Check sheet for the modelled part. Datum: model origin and axes. Units: mm. A direction names the side the tool comes from. Give positions to 0.01 mm unless a question says otherwise; leave off trailing zeros. Write each loop counter-clockwise with the first axis right and the second up, starting at its lowest first coordinate (ties: lowest second). Pieces come first, ordered by that corner, then holes. Notation, with made-up numbers: (-32, -11) -> (-27, -11) arc R12 ccw to (-27, 7) -> close; hole circle Ø3 at (16, 38). An arc over 180 degrees is marked (long way). Return JSON: item names as keys, results as strings.
from build123d import *

# Parameters (mm, degrees)
F1_DEPTH  = 153.75
F2_SIZE   = 3
F3_R      = 3.1
F4_DEPTH  = 11.001
F6_DEPTH  = 7
F7_R      = 27
F8_DEPTH  = 18.67
F9_R      = 14.75
F10_DEPTH = 3
F12_W     = 1
F12_H     = 1
F14_R     = 7.5
F15_DEPTH = 18.5
F16_R     = 9.425
F16_R_2   = 7.5
F17_DEPTH = 13.08
F19_DEPTH = 16
F20_R     = 27.5
F21_DEPTH = 10


# Not quite as in the source:
# - the program builds the solid bodies; features that only make, move or delete a surface that nothing else refers to are left out


with BuildPart() as f1:
    # F0 (on Front) → F1 (new body)
    with BuildSketch(Plane.XZ):
        Polygon((0, 11), (0, 0), (94, 0), (94, 11), (82, 11), (82, 77), (12, 77), (12, 11), align=None)
    extrude(amount=F1_DEPTH)

    # F2
    f2_edges = [f1.edges().sort_by_distance(p)[0] for p in [
        (12, -76.875, 77),
        (82, -76.875, 77),
    ]]
    chamfer(f2_edges, length=F2_SIZE)

    # F3 (on face) → F4 (cut, through all)
    with BuildSketch(Plane.XY.offset(11)):
        with Locations((89, -133.75)):
            Circle(F3_R)
        with Locations((89, -95.65)):
            Circle(F3_R)
        with Locations((89, -57.55)):
            Circle(F3_R)
        with Locations((89, -19.45)):
            Circle(F3_R)
        with Locations((5, -19.45)):
            Circle(F3_R)
        with Locations((5, -57.55)):
            Circle(F3_R)
        with Locations((5, -95.65)):
            Circle(F3_R)
        with Locations((5, -133.75)):
            Circle(F3_R)
    extrude(amount=-F4_DEPTH, mode=Mode.SUBTRACT)

    # F5 (on face) → F6 (join)
    with BuildSketch(Plane.XZ.offset(153.75)):
        with BuildLine():
            Line((25.9310321962, 77), (25.9310321962, 62.0646068434))
            ThreePointArc((25.9310321962, 62.0646068434), (15.39, 38.5), (25.9310321962, 14.9353931566))
            Line((25.9310321962, 14.9353931566), (25.9310321962, 0))
            Line((25.9310321962, 0), (68.0689678038, 0))
            Line((68.0689678038, 0), (68.0689678038, 14.9353931566))
            ThreePointArc((68.0689678038, 14.9353931566), (78.61, 38.5), (68.0689678038, 62.0646068434))
            Line((68.0689678038, 62.0646068434), (68.0689678038, 77))
            Line((68.0689678038, 77), (25.9310321962, 77))
        make_face()
    extrude(amount=F6_DEPTH)

    # F7 (on face) → F8 (join)
    with BuildSketch(Plane.XZ.offset(160.75)):
        with Locations((47, 38.5)):
            Circle(F7_R)
    extrude(amount=F8_DEPTH)

    # F9 (on face) → F10 (join)
    with BuildSketch(Plane.XZ.offset(179.42)):
        with Locations((47, 38.5)):
            Circle(F9_R)
    extrude(amount=F10_DEPTH)

    # F12 (on offset) → F13 (revolve, cut)
    with BuildSketch(Plane.YZ.offset(47)):
        with Locations((-170.5, 65)):
            Rectangle(F12_W, F12_H)
    revolve(axis=Axis((47, -160.75, 38.5), (0, 1, 0)), mode=Mode.SUBTRACT)

    # F14 (on face) → F15 (join)
    with BuildSketch(Plane.XZ.offset(182.42)):
        with Locations((47, 38.5)):
            Circle(F14_R)
    extrude(amount=F15_DEPTH)

    # F16 (on face) → F17 (join)
    with BuildSketch(Plane.XZ.offset(200.92)):
        with Locations((47, 38.5)):
            Circle(F16_R)
        with Locations((47, 38.5)):
            Circle(F16_R_2, mode=Mode.SUBTRACT)
        with Locations((47, 38.5)):
            Circle(F16_R_2)
    extrude(amount=F17_DEPTH)

    # F18 (on face) → F19 (join)
    with BuildSketch(Plane(origin=(0, 0, 0), x_dir=(-1, 0, 0), z_dir=(0, 1, 0))):
        Polygon((-79, 77), (-82, 74), (-82, 0), (-12, 0), (-12, 74), (-15, 77), align=None)
    extrude(amount=F19_DEPTH)

    # F20 (on face) → F21 (join)
    with BuildSketch(Plane(origin=(0, 16, 0), x_dir=(-1, 0, 0), z_dir=(0, 1, 0))):
        with Locations((-47, 38.5)):
            Circle(F20_R)
    extrude(amount=F21_DEPTH)


solid = f1.part
(1) Thickness scan on L1, parallel to Y at x = 89, z = 3; L2, parallel to X at y = -133.75, z = 3.25; L3, parallel to X at y = -133, z = 7. Record the ranges inside material, lowest first.
Reply:
{"L1": "-153.75 to -136.85, -130.65 to -98.75, -92.55 to -60.65, -54.45 to -22.55, -16.35 to 0", "L2": "0 to 1.9, 8.1 to 85.9, 92.1 to 94", "L3": "0 to 1.99, 8.01 to 85.99, 92.01 to 94"}
(2) Set-up check for faces 4 (the flat face through (78, -153.75, 30)), 5 (the flat face through (59, -179.42, 27)), 6 (the flat face through (6, -76, 11)), 7 (the flat face through (88, 0, 6)): record each of +Z, -Z, +X, -X, +Y, -Y from which the full face is reachable in a straight line by a thin tool's end or side.
Reply:
{"face 4": "+X, -Y", "face 5": "-Y", "face 6": "+Z, -X, +Y, -Y", "face 7": "+Z, -Z, +X, +Y"}
(3) Cross-section at C-C on y = -103. Enter the section's corners in (x, z).
Reply:
{"outline": "(0, 0) -> (94, 0) -> (94, 11) -> (82, 11) -> (82, 74) -> (79, 77) -> (15, 77) -> (12, 74) -> (12, 11) -> (0, 11) -> close"}
(4) Depth check by flat-ended pin: pin 1 Ø13 at (x, y) = (4.5, -114) entering from +Z; pin 2 Ø6 at (y, z) = (-156.5, 56) entering from +X; pin 3 Ø6 at (x, z) = (55.5, 50) entering from -Y; pin 4 Ø2 at (x, y) = (60, -75.5) entering from -Z. Enter the tip coordinate at first touch or a pass-through.
Reply:
{"pin 1": "z = 11", "pin 2": "x = 82", "pin 3": "y = -182.42", "pin 4": "z = 0"}
(5) Cross-section at B-B on y = -19.45. Enter the section's corners in (x, z).
Reply:
{"outline": "(0, 0) -> (1.9, 0) -> (1.9, 11) -> (0, 11) -> close; (8.1, 0) -> (85.9, 0) -> (85.9, 11) -> (82, 11) -> (82, 74) -> (79, 77) -> (15, 77) -> (12, 74) -> (12, 11) -> (8.1, 11) -> close; (92.1, 0) -> (94, 0) -> (94, 11) -> (92.1, 11) -> close"}
(6) Cross-section at A-A on x = 89. Enter the section's corners in (y, z), then the cut area to 3 significant figures.
Reply:
{"outline": "(-153.75, 0) -> (-136.85, 0) -> (-136.85, 11) -> (-153.75, 11) -> close; (-130.65, 0) -> (-98.75, 0) -> (-98.75, 11) -> (-130.65, 11) -> close; (-92.55, 0) -> (-60.65, 0) -> (-60.65, 11) -> (-92.55, 11) -> close; (-54.45, 0) -> (-22.55, 0) -> (-22.55, 11) -> (-54.45, 11) -> close; (-16.35, 0) -> (0, 0) -> (0, 11) -> (-16.35, 11) -> close", "area": "1,420 mm^2"}
(7) Release check for a two-part mould opening along X. For faces 1 (the flat face through (0, -76, 6)), 2 (the flat face through (69, -171, 53)), 3 (the cylindrical face through (4.596, -130.676, 5.577)) record: pulls with the +X half, pulls with the -X half, needs draft (parallel to the pull), parting line crosses it, or undercut.
Reply:
{"face 1": "pulls with the -X half", "face 2": "needs draft", "face 3": "undercut"}
